from build123d import *

# Parameters (mm, degrees)
ESQUISSE1_R        = 1.5
BOSS_EXTRU_1_DEPTH = 5


with BuildPart() as part:
    # Esquisse1 → Boss.-Extru.1 (new body)
    with BuildSketch(Plane.XY):
        with BuildLine():
            Line((0, 8), (20, 8))
            Line((20, 8), (32.728942549, 8))
            ThreePointArc((32.728942549, 8), (58.84637819, 0.211993808), (82.631578947, 13.517545651))
            ThreePointArc((82.631578947, 13.517545651), (86.714862069, 14.137746418), (87.547938522, 10.092522856))
            ThreePointArc((87.547938522, 10.092522856), (73.619262105, -3.172854276), (55, -8))
            Line((55, -8), (0, -8))
            Line((0, -8), (-20, -8))
            ThreePointArc((-20, -8), (-28, 0), (-20, 8))
            Line((-20, 8), (0, 8))
        make_face()
        Circle(ESQUISSE1_R, mode=Mode.SUBTRACT)
        with Locations((-20, 0)):
            Circle(ESQUISSE1_R, mode=Mode.SUBTRACT)
    extrude(amount=BOSS_EXTRU_1_DEPTH)


solid = part.part
Design review of the part built by this model. Coordinates are the model's own, in mm. Round coordinates to 2 decimals unless told otherwise and drop trailing zeros. Write each loop counter-clockwise with the first axis right and the second up, starting at its lowest first coordinate (ties: lowest second). Pieces come first, ordered by that corner, then holes. Notation, with made-up numbers: (-37, -30.75) -> (21, -30.75) arc R18 cw to (21, -16.75) -> close; hole circle Ø6 at (36, 1.5). An arc over 180 degrees is marked (long way). One line per question, with ' | ' between items.
(1) Take a section at D-D, the plane x = 28.5. State the section outline as (y, z) points, and give its area (3 significant figures).
Result sheet:
outline: (-8, 0) -> (8, 0) -> (8, 5) -> (-8, 5) -> close | area: 80.0 mm2
(2) Draft analysis for pull direction X (two halves, no side actions). For faces 1 (the flat face through (6, 8, 2)), 2 (the cylindrical face through (58.46, 0.17, 2.46)), 3 (the cylindrical face through (-28, 0, 2)), state which applies: released by +X, released by -X, zero draft, split by the parting line, or undercut.
Result sheet:
face 1: zero draft | face 2: undercut | face 3: released by -X
(3) Take a section at A-A, the plane z = 1.8. State the section outline as (x, y) points.
Result sheet:
outline: (-20, -8) -> (55, -8) arc R38.32 ccw to (87.55, 10.09) arc R3 ccw to (82.63, 13.52) arc R35 cw to (32.73, 8) -> (-20, 8) arc R8 ccw to start; hole circle Ø3 at (-20, 0); hole circle Ø3 at (0, 0)
(4) Take a section at B-B, the plane x = 0. State the section outline as (y, z) points, and give its area (3 significant figures).
Result sheet:
outline: (-8, 0) -> (-1.5, 0) -> (-1.5, 5) -> (-8, 5) -> close; (1.5, 0) -> (8, 0) -> (8, 5) -> (1.5, 5) -> close | area: 65.0 mm2
(5) Take a section at C-C, the plane y = 6.75. State the section outline as (x, z) points, and give its area (3 significant figures).
Result sheet:
outline: (-24.29, 0) -> (34.34, 0) -> (34.34, 5) -> (-24.29, 5) -> close; (75.66, 0) -> (85.22, 0) -> (85.22, 5) -> (75.66, 5) -> close | area: 341 mm2
(6) Insertion check: P1, Ø1, axis at y = 6, z = 2.5, coming from the +X side; P2, Ø2.5, axis at x = -5.5, z = 3.5, coming from the +Y side; P3, Ø3, axis at x = 46.5, z = 1, coming from the +Y side. Each pin has a flat end and moves straight along its axis. Give the tip position at first contact, or say it passes through.
Result sheet:
P1: x = 85.02 | P2: y = 8 | P3: y = 1.46
(7) Wall thickness on line 1 (Y direction, x = -20, z = 1.4); line 2 (X direction, y = -0.25, z = 2.95); line 3 (X direction, y = 5.75, z = 3.2): over which ranges is each line inside the solid? List them lowest first. Write a range as [from, to].
Result sheet:
line 1: [-8, -1.5], [1.5, 8] | line 2: [-28, -21.48], [-18.52, -1.48], [1.48, 78.11] | line 3: [-25.56, 35.78], [74.22, 84.41]
